from build123d import *

# Parameters (mm, degrees)
CHAMFER1_SIZE      = 0.5
CHAMFER1_SIZE2     = 0.866025404
CUT_EXTRUDE1_START = -13.35
SKETCH2_OUTSIDE_W  = 23.328
SKETCH2_OUTSIDE_H  = 23.328
SKETCH2_OUTSIDE_R  = 2.75
CUT_EXTRUDE1_DEPTH = 1


with BuildPart() as part:
    # Sketch1 → Revolve1 (revolve)
    with BuildSketch(Plane(origin=(0, 0, 0), x_dir=(0, 0, -1), z_dir=(1, 0, 0)), mode=Mode.PRIVATE) as revolve1_sk:
        Polygon((-36, 0), (-36, 3.4), (2.432191781, 3.4), (36, 3.4), (36, 0), align=None)
    revolve(revolve1_sk.sketch.rotate(Axis((0, 0, 36), (0, 0, -1)), 180), axis=Axis((0, 0, 36), (0, 0, -1)))

    # Chamfer1
    chamfer1_edges = [part.edges().sort_by_distance(p)[0] for p in [
        (0, 3.4, -36),
        (0, 3.4, 36),
    ]]
    chamfer1_side = [part.faces().sort_by_distance(p)[0] for p in [
        (0, 3.4, 0),
    ]]
    chamfer(chamfer1_edges, length=CHAMFER1_SIZE, length2=CHAMFER1_SIZE2, reference=chamfer1_side[0])

    # Sketch2 outside → Cut-Extrude1 (cut)
    with BuildSketch(Plane(origin=(0, 0, -36), x_dir=(-1, 0, 0), z_dir=(0, 0, -1)).offset(CUT_EXTRUDE1_START)):
        Rectangle(SKETCH2_OUTSIDE_W, SKETCH2_OUTSIDE_H)
        Circle(SKETCH2_OUTSIDE_R, mode=Mode.SUBTRACT)
    cut_extrude1 = extrude(amount=-CUT_EXTRUDE1_DEPTH, mode=Mode.SUBTRACT)

    # Mirror1: Cut-Extrude1 across plane
    add(cut_extrude1.mirror(Plane.XY), mode=Mode.SUBTRACT)


solid = part.part
Geometry check sheet. Reference: the model listing, model coordinates, mm. A direction names the side the tool comes from. Round coordinates to 2 decimals unless told otherwise and drop trailing zeros. Order: outer loops, then holes, each group sorted by start corner. A loop starts at its lowest first (then second) coordinate and runs counter-clockwise, first axis right, second up. Notation, with made-up numbers: M 24,9.5 L 58,9.5 A13 cw 58,32.5 Z; hole C -24,-40 d8. An arc over 180 degrees is marked long. Answer in a Markdown table with one row per item.
(1) Tool access check on faces 1 (the face through (3.32, 0.74, 0.3)), 2 (the face through (-3, 0, -22.65)). Record the directions out of +Z, -Z, +X, -X, +Y, -Y that give a thin tool (end or side, any length) a straight path to the whole face; none if there is none.
Responses:
| item | result |
|---|---|
| face 1 | +Z, -Z |
| face 2 | none |
(2) Sectioned sample at A-A, the plane z = 29. Record the cut outline in (x, y).
Responses:
| item | result |
|---|---|
| outline | C 0,0 d6.8 |
(3) Go/stop test with a flat-tipped pin: P1, Ø1.5, axis at y = -2.5, z = -3, coming from the +X side. Record where the tip stops, or that it passes through.
Responses:
| item | result |
|---|---|
| P1 | stops at x = 2.92 |
(4) Scan lines: probe 1 along Y at (x, z) = (2, 10); probe 2 along Z at (x, y) = (-0.5, -2.5); probe 3 along Z at (x, y) = (-1.5, 2.5). Record each from-to range of solid material in increasing order. Write a range as from..to.
Responses:
| item | result |
|---|---|
| probe 1 | y = -2.75..2.75 |
| probe 2 | z = -35.99..35.99 |
| probe 3 | z = -35.78..-22.65, -21.65..21.65, 22.65..35.78 |
